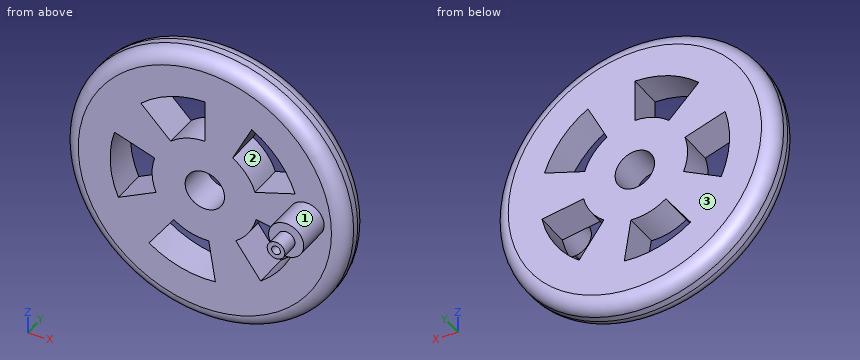
```python
from build123d import *

# Parameters (mm, degrees)
F0_R      = 25.4
F1_DEPTH  = 6.35
F2_R      = 2.54
F4_DEPTH  = 6.35
F6_D      = 7.112
F7_R      = 3.175
F8_DEPTH  = 6.35
F9_R      = 1.5875
F10_DEPTH = 3.175
F12_D     = 1.5875
F12_DEPTH = 6.35
F12_TIP   = 0.4769331164


with BuildPart() as f1:
    # F0 (on Front) → F1 (new body)
    with BuildSketch(Plane.XZ):
        Circle(F0_R)
    extrude(amount=F1_DEPTH)

    # F2
    f2_edges = [f1.edges().sort_by_distance(p)[0] for p in [
        (-25.4, -6.35, 0),
        (-25.4, 0, 0),
    ]]
    fillet(f2_edges, radius=F2_R)

    # F3 (on face) → F4 (cut)
    with BuildSketch(Plane.XZ.offset(6.35)):
        with BuildLine():
            ThreePointArc((-6.1549146928, 7.2692950225), (-3.2776203189, 8.9433120288), (0, 9.525))
            Line((0, 9.525), (0, 17.145))
            ThreePointArc((0, 17.145), (-6.1786433002, 15.9484075566), (-11.5430683654, 12.6574486952))
            Line((-11.5430683654, 12.6574486952), (-6.1549146928, 7.2692950225))
        make_face()
        with BuildLine():
            ThreePointArc((-8.8154836391, -3.6073360267), (-9.5184355619, -0.3535667594), (-9.0588133177, 2.9433868714))
            Line((-9.0588133177, 2.9433868714), (-16.3058639719, 5.2980963686))
            ThreePointArc((-16.3058639719, 5.2980963686), (-17.0771427132, -0.9479100044), (-15.6049533534, -7.0667436347))
            Line((-15.6049533534, -7.0667436347), (-8.8154836391, -3.6073360267))
        make_face()
        with BuildLine():
            Line((1.8986768002, -17.0249364512), (0.7066461766, -9.4987512959))
            ThreePointArc((0.7066461766, -9.4987512959), (-2.6050963781, -9.1618283034), (-5.5986545281, -7.7058868714))
            Line((-5.5986545281, -7.7058868714), (-10.0775781506, -13.8705963686))
            ThreePointArc((-10.0775781506, -13.8705963686), (-4.3756113272, -16.5342481576), (1.8986768002, -17.0249364512))
        make_face()
        with BuildLine():
            Line((16.7784001495, -3.4552457484), (9.2522149942, -2.2632151248))
            ThreePointArc((9.2522149942, -2.2632151248), (7.9083974563, -5.3087545312), (5.5986545281, -7.7058868714))
            Line((5.5986545281, -7.7058868714), (10.0775781506, -13.8705963686))
            ThreePointArc((10.0775781506, -13.8705963686), (14.3728661914, -9.2708173354), (16.7784001495, -3.4552457484))
        make_face()
        with BuildLine():
            ThreePointArc((5.0115371611, 8.1000074249), (7.4927548026, 5.8808375652), (9.0588133177, 2.9433868714))
            Line((9.0588133177, 2.9433868714), (16.3058639719, 5.2980963686))
            ThreePointArc((16.3058639719, 5.2980963686), (13.2585311493, 10.8045679408), (8.4709447691, 14.8894771392))
            Line((8.4709447691, 14.8894771392), (5.0115371611, 8.1000074249))
        make_face()
    extrude(amount=-F4_DEPTH, mode=Mode.SUBTRACT)

    # F6 (through all)
    with Locations(Plane.XZ.offset(6.35)):
        with Locations((0, 0)):
            Hole(F6_D / 2)

    # F7 (on face) → F8 (join)
    with BuildSketch(Plane.XZ.offset(6.35)):
        with Locations((18.3614359412, 1.1536982916)):
            Circle(F7_R)
    extrude(amount=F8_DEPTH)

    # F9 (on face) → F10 (join)
    with BuildSketch(Plane.XZ.offset(12.7)):
        with Locations((18.3614359412, 1.1536982916)):
            Circle(F9_R)
    extrude(amount=F10_DEPTH)

    # F12
    with Locations(Plane.XZ.offset(15.875)):
        with Locations((18.3614359412, 1.1536982916)):
            Hole(F12_D / 2, depth=F12_DEPTH)
            with Locations((0, 0, -(F12_DEPTH + F12_TIP / 2))):  # 118° drill point
                Cone(0, F12_D / 2, F12_TIP, mode=Mode.SUBTRACT)


solid = f1.part
```
The model under review builds one solid part; all positions refer to its coordinate system, in mm. Face numbers are marked on the shaded views. Give positions to 0.01 mm unless a question says otherwise; leave off trailing zeros. Write each loop counter-clockwise with the first axis right and the second up, starting at its lowest first coordinate (ties: lowest second). Pieces come first, ordered by that corner, then holes.
(1) Consider section A-A, the plane y = -1.5. Give the boundary of the cut face in (x, z) (3 decimals), and give its area (3 significant figures).
(2) The part is to be moulded in two halves that separate along X. For the marked faces 1, 2 and 3, say which applies: released by +X, released by -X, zero draft, split by the parting line, or undercut.
(3) For P1, Ø5, axis at x = 13.5, y = -8.5, coming from the +Z side; P2, Ø9, axis at x = 0, z = 0, coming from the +Y side; P3, Ø1.9, axis at y = -3.5, z = 14.5, coming from the -X side; P4, Ø5, axis at y = -14, z = 2.5, coming from the -X side, all flat-tipped, find the tip position at first contact; note any pin that passes through.
(4) Consider section B-B, the plane z = -4.5. Give the number of separate pieces and of enclosed holes in the cut face, and give its area (3 significant figures).
(5) To check wall thickness, follow L1, parallel to Y at x = -13.5, z = -16.5; L2, parallel to Z at x = -6.5, y = -2. State the ranges of each line that lie inside material, in increasing order.
Returned:
1. outline: circle Ø50.355 at (0, 0); hole (-16.306, 5.298) arc R17.626 ccw to (-15.605, -7.067) - (-8.815, -3.607) arc R9.525 cw to (-9.059, 2.943) - close; hole (-11.543, 12.657) - (-6.155, 7.269) arc R9.525 cw to (0, 9.525) - (0, 17.145) arc R17.626 ccw to start; hole (-10.078, -13.871) arc R17.626 ccw to (1.899, -17.025) - (0.707, -9.499) arc R9.525 cw to (-5.599, -7.706) - close; hole circle Ø7.112 at (0, 0); hole (5.012, 8.1) arc R9.525 cw to (9.059, 2.943) - (16.306, 5.298) arc R17.626 ccw to (8.471, 14.889) - close; hole (5.599, -7.706) - (10.078, -13.871) arc R17.626 ccw to (16.778, -3.455) - (9.252, -2.263) arc R9.525 cw to start
1. area: 1,580 mm2
2. face 1: split by the parting line
2. face 2: undercut
2. face 3: zero draft
3. P1: stops at z = 20.26
3. P2: stops at y = 0
3. P3: stops at x = -21.48
3. P4: stops at x = 15.19
4. separate pieces: 3
4. enclosed holes: 0
4. area: 223 mm2
5. L1: y = -6.35 to 0
5. L2: z = -24.49 to -15.83, -8.95 to 7.61, 15.82 to 24.49
